Here's how the part is built. I have some questions about the finished solid (model axes, mm). A direction names the side the tool comes from. Round coordinates to 2 decimals unless told otherwise and drop trailing zeros. Order: outer loops, then holes, each group sorted by start corner. A loop starts at its lowest first (then second) coordinate and runs counter-clockwise, first axis right, second up. Notation, with made-up numbers: M 89.25,2 L 141.25,2 A23 cw 141.25,19 Z; hole C -24,79.5 d4. An arc over 180 degrees is marked long. Write item = value, one per line. Start each with the question number.
Item 1: For faces 1 (the face through (1.68, -25.4, 0.53)), 2 (the face through (7.92, -31, 0)), 3 (the face through (-7.875, -31, 0)), 4 (the face through (6, -31, -1.11)), 5 (the face through (-5.695, -10.73, 5.493)), which set-ups out of +Z, -Z, +X, -X, +Y, -Y let a thin tool reach every point of the face, with its end or its side?
Item 2: I want a section at A-A, the plane y = 0. List the corners of the cut face in (x, z) for me.
Item 3: I'm going to push flat-ended pins straight in: P1, Ø0.5, axis at y = -9.5, z = 5.5, coming from the +X side; P2, Ø2, axis at y = -28.5, z = 4, coming from the +X side; P3, Ø0.5, axis at x = -10, z = 5.5, coming from the -Y side; P4, Ø1.5, axis at x = 1, y = 1, coming from the -Z side. Where does each tip first touch, or does it pass through?
Item 4: I want a section at B-B, the plane z = -3.25. List the corners of the cut face in (x, y) for me, plus the area to 3 significant figures.
Item 5: I want a section at D-D, the plane x = -20. List the corners of the cut face in (y, z) for me.
Item 6: We'd pull the mould along X, two halves only. Please class faces 6 (the face through (-11.35, -11.9, 5.5)), 7 (the face through (16.698, -12.839, 0.07)), 8 (the face through (1.69, -12.04, 5.49)), 9 (the face through (6, -12, 5)): pulls with the +X half, pulls with the -X half, needs draft (parallel to the pull), parting line crosses it, or undercut.
Item 7: Please list where these lines run through material, in increasing order: L1, parallel to Z at x = 11.5, y = -5; L2, parallel to Y at x = 4.5, z = 2.5; L3, parallel to X at y = 0.5, z = 4.25.
Item 8: I want a section at C-C, the plane y = -21. List the corners of the cut face in (x, z) for me, plus the area to 3 significant figures.
```python
from build123d import *

# Parameters (mm, degrees)
F0_R      = 3
F1_DEPTH  = 5
F2_R      = 1.7610809182
F3_DEPTH  = 15
F5_DEPTH  = 5
F6_W      = 22
F6_H      = 12
F7_DEPTH  = 1
F9_DEPTH  = 1
F10_DEPTH = 1


with BuildPart() as f1:
    # F0 (on Top) → F1 (new body, symmetric)
    with BuildSketch(Plane.XY):
        with BuildLine():
            Line((7.5, 6), (-7.5, 6))
            Line((-7.5, 6), (-21.2545811556, -1.0983172864))
            ThreePointArc((-21.2545811556, -1.0983172864), (-23.3778564167, -4.0725637723), (-22.1978447385, -7.5311780081))
            Line((-22.1978447385, -7.5311780081), (-11.3497786224, -18))
            Line((-11.3497786224, -18), (-5, -18))
            Line((-5, -18), (5, -18))
            Line((5, -18), (11.3497786224, -18))
            Line((11.3497786224, -18), (22.1978447385, -7.5311780081))
            ThreePointArc((22.1978447385, -7.5311780081), (23.3778564167, -4.0725637723), (21.2545811556, -1.0983172864))
            Line((21.2545811556, -1.0983172864), (7.5, 6))
        make_face()
        Circle(F0_R, mode=Mode.SUBTRACT)
    extrude(amount=F1_DEPTH, both=True)

    # F2 (on face) → F3 (join)
    with BuildSketch(Plane.XZ.offset(18)):
        with BuildLine():
            ThreePointArc((0, -5), (3.5355339059, -3.5355339059), (5, 0))
            ThreePointArc((5, 0), (3.5355339126, 3.5355338993), (1.89e-08, 5))
            ThreePointArc((1.89e-08, 5), (-5, 9.4e-09), (0, -5))
        make_face()
        Circle(F2_R, mode=Mode.SUBTRACT)
    extrude(amount=F3_DEPTH)

    # F4 (on face) → F5 (join)
    with BuildSketch(Plane.XZ.offset(33)):
        with BuildLine():
            Line((-7.8751421592, -1.1104003458), (-4.8751421592, -1.1104003458))
            ThreePointArc((-4.8751421592, -1.1104003458), (-4.9987302039, -0.1126780739), (-4.9202248379, 0.8895996542))
            Line((-4.9202248379, 0.8895996542), (-7.8751421592, 0.8895996542))
            Line((-7.8751421592, 0.8895996542), (-7.8751421592, -1.1104003458))
        make_face()
        with BuildLine():
            ThreePointArc((5, 0), (4.9800162745, -0.4465847123), (4.9202248379, -0.8895996542))
            Line((4.9202248379, -0.8895996542), (4.9202248379, -1.1104003458))
            Line((4.9202248379, -1.1104003458), (7.9202248379, -1.1104003458))
            Line((7.9202248379, -1.1104003458), (7.9202248379, 0.8895996542))
            Line((7.9202248379, 0.8895996542), (4.9202248379, 0.8895996542))
            ThreePointArc((4.9202248379, 0.8895996542), (4.9800162745, 0.4465847123), (5, 0))
        make_face()
    extrude(amount=-F5_DEPTH)

    # F6 (on face) → F7 (join)
    with BuildSketch(Plane(origin=(0, 0, -5), x_dir=(1, 0, 0), z_dir=(0, 0, -1))):
        with Locations((0.3497786224, 12)):
            Rectangle(F6_W, F6_H)
    extrude(amount=F7_DEPTH)

    # F8 (on face) → F9 (join)
    with BuildSketch(Plane.XY.offset(5)):
        Polygon((-11.3497786224, -6), (-11.3497786224, -18), (1.08e-08, -18), (10.6502213776, -18), (10.6502213776, -6), align=None)
        with BuildLine():
            Line((-6.5919761548, -13.2537334136), (-4.7731608238, -8.1352665147))
            Line((-4.7731608238, -8.1352665147), (-3.7783873047, -8.1352665147))
            Line((-3.7783873047, -8.1352665147), (-6.6459831235, -16.0951968282))
            Line((-6.6459831235, -16.0951968282), (-7.5606172698, -16.0951968282))
            Line((-7.5606172698, -16.0951968282), (-10.4142758064, -8.1352665147))
            Line((-10.4142758064, -8.1352665147), (-9.4334395695, -8.1352665147))
            Line((-9.4334395695, -8.1352665147), (-7.6041712768, -13.2850922986))
            add(Edge.make_bspline(
                [(-7.6041712768, -13.2850922986), (-7.2888402663, -14.1735940408), (-7.1041712768, -15.0115731349)],
                knots=[0, 0, 0, 1, 1, 1], degree=2))
            add(Edge.make_bspline(
                [(-7.1041712768, -15.0115731349), (-6.9073071653, -14.1300400338), (-6.5919761548, -13.2537334136)],
                knots=[0, 0, 0, 1, 1, 1], degree=2))
        make_face(mode=Mode.SUBTRACT)
        Polygon((3.2773618243, -16.0951968282), (2.319173671, -16.0951968282), (1.3278844723, -13.5638379432), (-1.862010998, -13.5638379432), (-2.8411050747, -16.0951968282), (-3.7783873047, -16.0951968282), (-0.6320458412, -8.1021654694), (0.1466998034, -8.1021654694), align=None, mode=Mode.SUBTRACT)
        with BuildLine():
            add(Edge.make_bspline(
                [(8.3923444027, -12.6492037969), (8.8627276779, -13.1613989188), (8.8627276779, -13.9767299293)],
                knots=[0, 0, 0, 1, 1, 1], degree=2))
            add(Edge.make_bspline(
                [(8.8627276779, -13.9767299293), (8.8627276779, -15.0272525774), (8.100532556, -15.6161027516)],
                knots=[0, 0, 0, 1, 1, 1], degree=2))
            add(Edge.make_bspline(
                [(8.100532556, -15.6161027516), (7.338337434, -16.2049529258), (6.031717225, -16.2049529258)],
                knots=[0, 0, 0, 1, 1, 1], degree=2))
            add(Edge.make_bspline(
                [(6.031717225, -16.2049529258), (4.6170830786, -16.2049529258), (3.8540168765, -15.8390992673)],
                knots=[0, 0, 0, 1, 1, 1], degree=2))
            Line((3.8540168765, -15.8390992673), (3.8540168765, -14.9471132046))
            add(Edge.make_bspline(
                [(3.8540168765, -14.9471132046), (4.3453060751, -15.1526881174), (4.9219611274, -15.2728971767)],
                knots=[0, 0, 0, 1, 1, 1], degree=2))
            add(Edge.make_bspline(
                [(4.9219611274, -15.2728971767), (5.4986161797, -15.3931062359), (6.0648182703, -15.3931062359)],
                knots=[0, 0, 0, 1, 1, 1], degree=2))
            add(Edge.make_bspline(
                [(6.0648182703, -15.3931062359), (6.9899053783, -15.3931062359), (7.4585464933, -15.0420609397)],
                knots=[0, 0, 0, 1, 1, 1], degree=2))
            add(Edge.make_bspline(
                [(7.4585464933, -15.0420609397), (7.9271876082, -14.6910156436), (7.9271876082, -14.0638379432)],
                knots=[0, 0, 0, 1, 1, 1], degree=2))
            add(Edge.make_bspline(
                [(7.9271876082, -14.0638379432), (7.9271876082, -13.6509459572), (7.7608113016, -13.3870086749)],
                knots=[0, 0, 0, 1, 1, 1], degree=2))
            add(Edge.make_bspline(
                [(7.7608113016, -13.3870086749), (7.594434995, -13.1230713927), (7.2050621727, -12.8992037969)],
                knots=[0, 0, 0, 1, 1, 1], degree=2))
            add(Edge.make_bspline(
                [(7.2050621727, -12.8992037969), (6.8156893504, -12.6753362011), (6.0212642633, -12.3931062359)],
                knots=[0, 0, 0, 1, 1, 1], degree=2))
            add(Edge.make_bspline(
                [(6.0212642633, -12.3931062359), (4.9115081657, -11.9958936924), (4.4350273295, -11.4514686052)],
                knots=[0, 0, 0, 1, 1, 1], degree=2))
            add(Edge.make_bspline(
                [(4.4350273295, -11.4514686052), (3.9585464933, -10.9070435181), (3.9585464933, -10.0307368979)],
                knots=[0, 0, 0, 1, 1, 1], degree=2))
            add(Edge.make_bspline(
                [(3.9585464933, -10.0307368979), (3.9585464933, -9.1108762708), (4.6493130438, -8.5664511836)],
                knots=[0, 0, 0, 1, 1, 1], degree=2))
            add(Edge.make_bspline(
                [(4.6493130438, -8.5664511836), (5.3400795943, -8.0220260965), (6.4794524166, -8.0220260965)],
                knots=[0, 0, 0, 1, 1, 1], degree=2))
            add(Edge.make_bspline(
                [(6.4794524166, -8.0220260965), (7.6658635664, -8.0220260965), (8.6623792459, -8.4575661662)],
                knots=[0, 0, 0, 1, 1, 1], degree=2))
            Line((8.6623792459, -8.4575661662), (8.3731806396, -9.262444215))
            add(Edge.make_bspline(
                [(8.3731806396, -9.262444215), (7.3871179218, -8.8495522289), (6.456804333, -8.8495522289)],
                knots=[0, 0, 0, 1, 1, 1], degree=2))
            add(Edge.make_bspline(
                [(6.456804333, -8.8495522289), (5.7216126953, -8.8495522289), (5.3078496291, -9.1648832394)],
                knots=[0, 0, 0, 1, 1, 1], degree=2))
            add(Edge.make_bspline(
                [(5.3078496291, -9.1648832394), (4.8940865629, -9.4802142498), (4.8940865629, -10.0411898596)],
                knots=[0, 0, 0, 1, 1, 1], degree=2))
            add(Edge.make_bspline(
                [(4.8940865629, -10.0411898596), (4.8940865629, -10.4540818457), (5.0465255873, -10.718890208)],
                knots=[0, 0, 0, 1, 1, 1], degree=2))
            add(Edge.make_bspline(
                [(5.0465255873, -10.718890208), (5.1989646117, -10.9836985704), (5.5613339497, -11.2040818457)],
                knots=[0, 0, 0, 1, 1, 1], degree=2))
            add(Edge.make_bspline(
                [(5.5613339497, -11.2040818457), (5.9237032877, -11.4244651209), (6.669347887, -11.6910156436)],
                knots=[0, 0, 0, 1, 1, 1], degree=2))
            add(Edge.make_bspline(
                [(6.669347887, -11.6910156436), (7.9219611274, -12.1370086749), (8.3923444027, -12.6492037969)],
                knots=[0, 0, 0, 1, 1, 1], degree=2))
        make_face(mode=Mode.SUBTRACT)
    extrude(amount=F9_DEPTH)

    # F8 (on face) → F10 (join)
    with BuildSketch(Plane.XY.offset(5)):
        with BuildLine():
            Line((-1.5344848656, -12.73108533), (1.0404280264, -12.73108533))
            Line((1.0404280264, -12.73108533), (0.1135987581, -10.2641863753))
            add(Edge.make_bspline(
                [(0.1135987581, -10.2641863753), (-0.0658437506, -9.7955452603), (-0.255739221, -9.1161027516)],
                knots=[0, 0, 0, 1, 1, 1], degree=2))
            add(Edge.make_bspline(
                [(-0.255739221, -9.1161027516), (-0.3759482803, -9.6387508352), (-0.5989447959, -10.2641863753)],
                knots=[0, 0, 0, 1, 1, 1], degree=2))
            Line((-0.5989447959, -10.2641863753), (-1.5344848656, -12.73108533))
        make_face()
    extrude(amount=F10_DEPTH)


solid = f1.part
```
Filled in:
q1.face_1 = -Y
q1.face_2 = +Z, -Z, +X, -Y
q1.face_3 = +Z, -Z, -X, -Y
q1.face_4 = -Z, +X, -Y
q1.face_5 = +Z
q2.outline = M -19.13,-5 L -3,-5 L -3,5 L -19.13,5 Z; M 3,-5 L 19.13,-5 L 19.13,5 L 3,5 Z
q3.P1 = 10.65
q3.P2 = 4
q3.P3 = -18
q3.P4 = through
q4.outline = M -22.2,-7.53 L -11.35,-18 L -3.8,-18 L -3.8,-33 L 3.8,-33 L 3.8,-18 L 11.35,-18 L 22.2,-7.53 A4 ccw 21.25,-1.1 L 7.5,6 L -7.5,6 L -21.25,-1.1 A4 ccw Z; hole C 0,0 d6
q4.area = 936 mm^2
q5.outline = M -9.65,-5 L -0.45,-5 L -0.45,5 L -9.65,5 Z
q6.face_6 = pulls with the -X half
q6.face_7 = pulls with the +X half
q6.face_8 = undercut
q6.face_9 = undercut
q7.L1 = -5 to 5
q7.L2 = -18 to 6
q7.L3 = -18.16 to -2.96, 2.96 to 18.16
q8.outline = C 0,0 d10; hole C 0,0 d3.52
q8.area = 68.8 mm^2
